Check sheet for the modelled part. Datum: model origin and axes. Units: mm. A direction names the side the tool comes from. Give positions to 0.01 mm unless a question says otherwise; leave off trailing zeros. Loops run counter-clockwise (first coordinate to the right, second up) from the corner with the lowest first, then second, coordinate; pieces in that order, holes last. Notation, with made-up numbers: (35, 77.25) -> (42, 77.25) arc R23 cw to (42, 112.25) -> close; hole circle Ø3 at (-28, 81.25). An arc over 180 degrees is marked (long way). Write each question's results on one line, items separated by ' | '. Start each with the question number.
Item 1: Access from +Z, -Z, +X, -X, +Y, -Y to the whole of each face (thin tool, end or side, straight path). Record for faces 5 (the face through (9, 3, -29)), 6 (the face through (17.38, 4.47, 24.56)), 7 (the face through (13.88, 6.14, -29.1)).
Item 2: Cross-section at B-B on x = -9. Enter the section's corners in (y, z), then the cut area to 3 significant figures.
Item 3: Mould release check, pull along Z, two halves, no side actions. Record for faces 1 (the face through (22, 3.25, 20)), 2 (the face through (25.408, 2.028, -23.707)), 3 (the face through (-22, 2, 28)), 4 (the face through (-6.2, 6.8, 7.1)): pulls with the +Z half, pulls with the -Z half, needs draft (parallel to the pull), parting line crosses it, or undercut.
Item 4: Cross-section at C-C on x = -17. Enter the section's corners in (y, z), then the cut area to 3 significant figures.
Item 5: Gauge pin test, flat ends, axial feed: pin 1 Ø2 at (x, y) = (12.5, 2.5) entering from -Z; pin 2 Ø12 at (x, z) = (1.5, -17) entering from -Y; pin 3 Ø0.6 at (y, z) = (7, 3) entering from -X. Record the tip position at first contact, or that the pin passes through.
Item 6: Scan lines: line 1 along X through (y, z) = (3.5, -25.75); line 2 along X through (y, z) = (4, 3.5); line 3 along X through (y, z) = (4.5, -32). Record each from-to range of solid material in increasing order.
Item 7: Cross-section at A-A on z = 4. Enter the section's corners in (x, y).
from build123d import *

# Parameters (mm, degrees)
BOSS_EXTRUDE1_DEPTH = 7
SKETCH2_W           = 43.5
SKETCH2_H           = 41.5
CUT_EXTRUDE1_DEPTH  = 6.25
BOSS_EXTRUDE2_DEPTH = 3
SKETCH4_W           = 43.25
SKETCH4_H           = 16.326941356
CUT_EXTRUDE2_DEPTH  = 2.5
SKETCH5_R           = 1.25
CUT_EXTRUDE3_DEPTH  = 6.5
SKETCH6_W           = 43.5
SKETCH6_H           = 41.5
SKETCH6_W_2         = 7
SKETCH6_H_2         = 7
BOSS_EXTRUDE3_DEPTH = 0.75
SKETCH7_W           = 41.285529239
SKETCH7_H           = 40.12964718
SKETCH7_W_2         = 37.285529239
SKETCH7_H_2         = 36.12964718
CUT_EXTRUDE4_DEPTH  = 0.5
CHAMFER1_SIZE       = 4
CHAMFER1_SIZE2      = 3.356398525
FILLET1_R           = 8
FILLET2_R           = 3
FILLET3_R           = 5
FILLET4_R           = 6.5
BOSS_EXTRUDE4_REACH = 42.311
SKETCH11_W          = 33
SKETCH11_H          = 13.592640687
CHAMFER2_SIZE       = 3.6
CHAMFER2_SIZE2      = 3.020758672
CUT_EXTRUDE7_START  = -5.5
SKETCH12_W          = 29
SKETCH12_H          = 17.85
CUT_EXTRUDE7_DEPTH  = 5.5


with BuildPart() as part:
    # Sketch1 → Boss-Extrude1 (new body)
    with BuildSketch(Plane(origin=(0, 0, 0), x_dir=(1, 0, 0), z_dir=(0, 1, 0))):
        Polygon((-26, 24), (-20, 30), (20, 30), (26, 24), (26, -24), (20, -30), (-20, -30), (-26, -24), align=None)
    extrude(amount=BOSS_EXTRUDE1_DEPTH)

    # Sketch2 → Cut-Extrude1 (cut)
    with BuildSketch(Plane.XZ):
        with Locations((1.75, 1.25)):
            Rectangle(SKETCH2_W, SKETCH2_H)
    extrude(amount=-CUT_EXTRUDE1_DEPTH, mode=Mode.SUBTRACT)

    # Sketch3 → Boss-Extrude2 (add)
    with BuildSketch(Plane.XZ.offset(-6.25)):
        Polygon((-20, 16), (-14, 22), (-20, 22), align=None)
        Polygon((-20, -13.5), (-14, -19.5), (-20, -19.5), align=None)
        Polygon((17.5, -19.5), (23.5, -19.5), (23.5, -13.5), align=None)
        Polygon((17.5, 22), (23.5, 16), (23.5, 22), align=None)
    extrude(amount=BOSS_EXTRUDE2_DEPTH)

    # Sketch4 → Cut-Extrude2 (cut)
    with BuildSketch(Plane.XZ):
        with Locations((0.125, 30.163470678)):
            Rectangle(SKETCH4_W, SKETCH4_H)
    extrude(amount=-CUT_EXTRUDE2_DEPTH, mode=Mode.SUBTRACT)

    # Sketch5 → Cut-Extrude3 (cut)
    with BuildSketch(Plane.XZ):
        with Locations(Location((-17, 25.75, 0), (0, 0, 270))):
            Circle(SKETCH5_R)
        with Locations(Location((17, 25.75, 0), (0, 0, 270))):
            Circle(SKETCH5_R)
        with Locations(Location((17, -25.75, 0), (0, 0, 270))):
            Circle(SKETCH5_R)
    extrude(amount=-CUT_EXTRUDE3_DEPTH, mode=Mode.SUBTRACT)

    # Sketch6 → Boss-Extrude3 (add)
    with BuildSketch(Plane.XZ.offset(-6.25)):
        with Locations((1.75, 1.25)):
            Rectangle(SKETCH6_W, SKETCH6_H)
        with Locations((12, -8)):
            Rectangle(SKETCH6_W_2, SKETCH6_H_2, mode=Mode.SUBTRACT)
    extrude(amount=BOSS_EXTRUDE3_DEPTH)

    # Sketch7 → Cut-Extrude4 (cut)
    with BuildSketch(Plane(origin=(0, 7, 0), x_dir=(1, 0, 0), z_dir=(0, 1, 0))):
        with Locations((0.35723538, -1.609430965)):
            Rectangle(SKETCH7_W, SKETCH7_H)
        with Locations((0.35723538, -1.609430965)):
            Rectangle(SKETCH7_W_2, SKETCH7_H_2, mode=Mode.SUBTRACT)
        with BuildLine():
            ThreePointArc((-13.273830834, 8.523353213), (-5.99678776, -7.326911946), (9.055555556, -16.136748619))
            ThreePointArc((9.055555556, -16.136748619), (10.851382953, -15.007587888), (9.722222222, -13.21176049))
            ThreePointArc((9.722222222, -13.21176049), (-3.77298213, -5.313286231), (-10.297227644, 8.897296325))
            ThreePointArc((-10.297227644, 8.897296325), (-11.972500795, 10.198626364), (-13.273830834, 8.523353213))
        make_face()
        with BuildLine():
            ThreePointArc((-6.328423391, 9.395887141), (-0.807907956, -2.628451945), (10.611111111, -9.311776318))
            ThreePointArc((10.611111111, -9.311776318), (12.406938509, -8.182615587), (11.277777778, -6.386788189))
            ThreePointArc((11.277777778, -6.386788189), (1.415897675, -0.61482623), (-3.351820202, 9.769830253))
            ThreePointArc((-3.351820202, 9.769830253), (-5.027093352, 11.071160292), (-6.328423391, 9.395887141))
        make_face()
        with BuildLine():
            ThreePointArc((0.616984051, 10.268421069), (4.380971848, 2.070008056), (12.166666667, -2.486804017))
            ThreePointArc((12.166666667, -2.486804017), (13.962494065, -1.357643286), (12.833333333, 0.438184112))
            ThreePointArc((12.833333333, 0.438184112), (6.604777479, 4.08363377), (3.593587241, 10.642364181))
            ThreePointArc((3.593587241, 10.642364181), (1.91831409, 11.94369422), (0.616984051, 10.268421069))
        make_face()
    extrude(amount=-CUT_EXTRUDE4_DEPTH, mode=Mode.SUBTRACT)

    # Chamfer1
    chamfer1_edges = [part.edges().sort_by_distance(p)[0] for p in [
        (0, 7, 30),
    ]]
    chamfer1_side = [part.faces().sort_by_distance(p)[0] for p in [
        (0, 4.75, 30),
    ]]
    chamfer(chamfer1_edges, length=CHAMFER1_SIZE, length2=CHAMFER1_SIZE2, reference=chamfer1_side[0])

    # Fillet1
    fillet1_edges = [part.edges().sort_by_distance(p)[0] for p in [
        (-26, 3.5, -24),
        (-20, 3.5, -30),
        (20, 3.5, -30),
        (26, 3.5, -24),
        (26, 3.5, 24),
        (-26, 3.5, 24),
    ]]
    fillet(fillet1_edges, radius=FILLET1_R)

    # Fillet2
    fillet2_edges = [part.edges().sort_by_distance(p)[0] for p in [
        (23.506626387, 7, 26.493373613),
        (0, 7, -30),
        (23, 7, -27),
        (-23.506626387, 7, 26.493373613),
        (26, 7, 0),
        (-23, 7, -27),
        (-26, 7, 0),
        (-25.39103626, 7, 23.74775896),
        (-25.39103626, 7, -23.74775896),
        (-19.74775896, 7, -29.39103626),
        (25.39103626, 7, 23.74775896),
        (25.39103626, 7, -23.74775896),
        (19.74775896, 7, -29.39103626),
    ]]
    fillet(fillet2_edges, radius=FILLET2_R)

    # Fillet3
    fillet3_edges = [part.edges().sort_by_distance(p)[0] for p in [
        (19, 6.75, -16.455392625),
        (-18.285529239, 6.75, -16.455392625),
        (-18.285529239, 6.75, 19.674254555),
        (19, 6.75, 19.674254555),
    ]]
    fillet(fillet3_edges, radius=FILLET3_R)

    # Fillet4
    fillet4_edges = [part.edges().sort_by_distance(p)[0] for p in [
        (-20.285529239, 6.75, 21.674254555),
        (-20.285529239, 6.75, -18.455392625),
        (21, 6.75, -18.455392625),
        (21, 6.75, 21.674254555),
    ]]
    fillet(fillet4_edges, radius=FILLET4_R)

    # Boss-Extrude4: up to this face of the body (flat: up to its plane)
    boss_extrude4_end = Plane(part.part.faces().sort_by_distance((-25.217296352, 0, 0))[0])
    # Sketch11 → Boss-Extrude4 (add, up to the picked face)
    with BuildSketch(Plane(origin=(0, 7, 0), x_dir=(1, 0, 0), z_dir=(0, 1, 0)), mode=Mode.PRIVATE) as boss_extrude4_sk1:
        with Locations((-5.5, 30.553679657)):
            Rectangle(SKETCH11_W, SKETCH11_H)
    boss_extrude4_tool1 = split(extrude(boss_extrude4_sk1.sketch, amount=-BOSS_EXTRUDE4_REACH, mode=Mode.PRIVATE), bisect_by=boss_extrude4_end, keep=Keep.BOTH, mode=Mode.PRIVATE)
    add(boss_extrude4_tool1.solids().sort_by(Axis((-5.5, 7, -30.55368), (0, -1, 0)))[0])

    # Chamfer2
    chamfer2_edges = [part.edges().sort_by_distance(p)[0] for p in [
        (-5.5, 7, -37.35),
    ]]
    chamfer2_side = [part.faces().sort_by_distance(p)[0] for p in [
        (-5.5, 3.5, -37.35),
    ]]
    chamfer(chamfer2_edges, length=CHAMFER2_SIZE, length2=CHAMFER2_SIZE2, reference=chamfer2_side[0])

    # Sketch12 → Cut-Extrude7 (cut)
    with BuildSketch(Plane.XZ.offset(CUT_EXTRUDE7_START)):
        with Locations((-5.5, -28.425)):
            Rectangle(SKETCH12_W, SKETCH12_H)
    extrude(amount=CUT_EXTRUDE7_DEPTH, mode=Mode.SUBTRACT)


solid = part.part
Answer sheet:
1) face 5: -Z, -Y | face 6: -Y | face 7: -Z, +X, +Y
2) outline: (2.5, 22) -> (5.5, 22) -> (5.5, -35.59) -> (7, -34.33) -> (7, -18.46) -> (6.5, -18.46) -> (6.5, -16.46) -> (7, -16.46) -> (7, -3.43) -> (6.5, -3.43) -> (6.5, 3.38) -> (7, 3.38) -> (7, 19.67) -> (6.5, 19.67) -> (6.5, 21.67) -> (7, 21.67) -> (7, 26.64) -> (3, 30) -> (2.5, 30) -> close | area: 109 mm²
3) face 1: undercut | face 2: pulls with the -Z half | face 3: pulls with the +Z half | face 4: undercut
4) outline: (2.5, 22) -> (3.25, 22) -> (3.25, 19) -> (5.5, 19) -> (5.5, -16.5) -> (3.25, -16.5) -> (3.25, -19.5) -> (5.5, -19.5) -> (5.5, -35.59) -> (7, -34.33) -> (7, -17.6) -> (6.5, -17.6) -> (6.5, -14.8) -> (7, -14.8) -> (7, 18.02) -> (6.5, 18.02) -> (6.5, 20.82) -> (7, 20.82) -> (7, 26.64) -> (3, 30) -> (2.5, 30) -> (2.5, 27) -> (6.5, 27) -> (6.5, 24.5) -> (2.5, 24.5) -> close | area: 115 mm²
5) pin 1: stops at z = -30 | pin 2: stops at y = 5.5 | pin 3: stops at x = -24.31
6) line 1: x = -24.19 to -20, 9 to 15.75, 18.25 to 24.19 | line 2: x = -26 to -20, 23.5 to 26 | line 3: x = -22 to -20, 9 to 11
7) outline: (-26, 0) -> (-20, 0) -> (-20, 5.5) -> (23.5, 5.5) -> (23.5, 0) -> (26, 0) -> (26, 4) arc R3 ccw to (23, 7) -> (21, 7) -> (21, 6.5) -> (19, 6.5) -> (19, 7) -> (5.47, 7) -> (5.47, 6.5) -> (0.55, 6.5) -> (0.55, 7) -> (-4.89, 7) -> (-4.89, 6.5) -> (-8.59, 6.5) -> (-8.59, 7) -> (-18.29, 7) -> (-18.29, 6.5) -> (-20.29, 6.5) -> (-20.29, 7) -> (-23, 7) arc R3 ccw to (-26, 4) -> close
